The drawing under review shows one solid part. Ordinate dimensions are in mm from its lowest x, y, z. A direction names the side the tool comes from. Coordinates: 2 decimals unless noted, no trailing zeros. Loops run counter-clockwise (first coordinate to the right, second up) from the corner with the lowest first, then second, coordinate; pieces in that order, holes last. Notation, with made-up numbers: (39.25, 57.5) - (48.25, 57.5) arc R19 ccw to (48.25, 89.5) - close; hole circle Ø9 at (6.5, -22). An arc over 180 degrees is marked (long way). Answer as a JSON object with one key per item and string values. Group by question number.
Item 1: We need section D-D (y = 79). Give the boundary of the cut face in (x, z).
Item 2: We need section C-C (x = 45.5). Give the boundary of the cut face in (y, z), then the cut area to 3 significant figures.
Item 3: We need section A-A (x = 64.5). Give the boundary of the cut face in (y, z), then the cut area to 3 significant figures.
Item 4: Clearance check with flat-ended pins moving along their axes: pin 1 (3 mm diameter, centred on y = 127.5, z = 33.5, fed in from +X); pin 2 (4 mm diameter, centred on x = 46.5, z = 10.5, fed in from +Y); pin 3 (10 mm diameter, centred on x = 29.5, y = 87, fed in from +Z). State where each tip first meets the part, or that it passes through.
Item 5: Mouldability with a two-part tool opening along Y and no side actions: class the marked faces 1, 2 and 3 as released by +Y, released by -Y, zero draft, split by the parting line, or undercut.
Item 6: To check wall thickness, follow line 1 (Y direction, x = 48, z = 31.5); line 2 (Y direction, x = 24, z = 4); line 3 (Y direction, x = 61.5, z = 53). State the ranges of each line that lie inside material, in increasing order.
Item 7: Tool access review of the marked faces 4 and 5: name each direction out of +Z, -Z, +X, -X, +Y, -Y from which nothing blocks a thin tool from reaching the whole face with its end or side.
Item 8: We need section B-B (z = 39.5). Give the boundary of the cut face in (x, y), then the cut area to 3 significant figures.
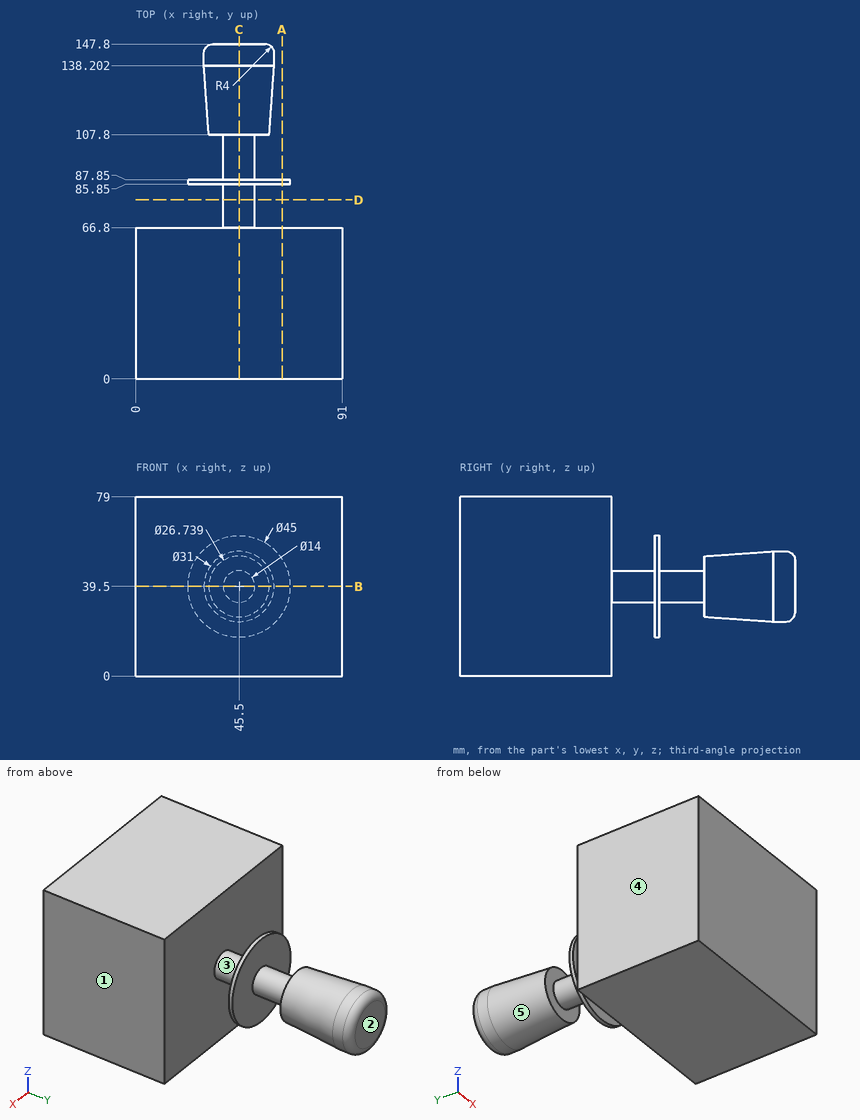
Check sheet entries:
{
 "1": {"outline": "circle Ø14 at (45.5, 39.5)"},
 "2": {"outline": "(0, 0) - (66.8, 0) - (66.8, 32.5) - (85.85, 32.5) - (85.85, 17) - (87.85, 17) - (87.85, 32.5) - (107.8, 32.5) - (107.8, 26.13) - (138.2, 24) - (143.8, 24) arc R4 ccw to (147.8, 28) - (147.8, 51) arc R4 ccw to (143.8, 55) - (138.2, 55) - (107.8, 52.87) - (107.8, 46.5) - (87.85, 46.5) - (87.85, 62) - (85.85, 62) - (85.85, 46.5) - (66.8, 46.5) - (66.8, 79) - (0, 79) - close", "area": "7,080 mm2"},
 "3": {"outline": "(0, 0) - (66.8, 0) - (66.8, 79) - (0, 79) - close; (85.85, 27.45) - (87.85, 27.45) - (87.85, 51.55) - (85.85, 51.55) - close", "area": "5,330 mm2"},
 "4": {"pin 1": "stops at x = 59.56", "pin 2": "stops at y = 66.8", "pin 3": "stops at z = 59.13"},
 "5": {"face 1": "zero draft", "face 2": "released by +Y", "face 3": "undercut"},
 "6": {"line 1": "y = 0 to 66.8, 85.85 to 87.85, 107.8 to 147.8", "line 2": "y = 0 to 66.8", "line 3": "y = 0 to 66.8, 85.85 to 87.85"},
 "7": {"face 4": "+Z, -Z, -X, +Y, -Y", "face 5": "none"},
 "8": {"outline": "(0, 0) - (91, 0) - (91, 66.8) - (52.5, 66.8) - (52.5, 85.85) - (68, 85.85) - (68, 87.85) - (52.5, 87.85) - (52.5, 107.8) - (58.87, 107.8) - (61, 138.2) - (61, 143.8) arc R4 ccw to (57, 147.8) - (34, 147.8) arc R4 ccw to (30, 143.8) - (30, 138.2) - (32.13, 107.8) - (38.5, 107.8) - (38.5, 87.85) - (23, 87.85) - (23, 85.85) - (38.5, 85.85) - (38.5, 66.8) - (0, 66.8) - close", "area": "7,880 mm2"}
}
